from build123d import *

# Parameters (mm, degrees)
BOSS_EXTRUDE1_DEPTH = 6


with BuildPart() as part:
    # Sketch1 → Boss-Extrude1 (new body)
    with BuildSketch(Plane.XY):
        with BuildLine():
            Line((0, 0), (0, 100))
            Line((0, 100), (0, 116.099356626))
            ThreePointArc((0, 116.099356626), (5.566363801, 126.764301673), (17.498623517, 128.296175326))
            Line((17.498623517, 128.296175326), (69.668134054, 109.054191593))
            ThreePointArc((69.668134054, 109.054191593), (74.638707981, 99.521504918), (65.633362838, 93.649326508))
            Line((65.633362838, 93.649326508), (38.741282829, 97.960661065))
            ThreePointArc((38.741282829, 97.960661065), (29.863968579, 95.470560576), (25.999999999, 87.099356626))
            Line((25.999999999, 87.099356626), (25.999999999, -325.14105767))
            ThreePointArc((25.999999999, -325.14105767), (26.999999698, -326.141057369), (27.999999397, -325.14105767))
            Line((27.999999397, -325.14105767), (27.999999397, -295.628663382))
            Line((27.999999397, -295.628663382), (29.999999399, -295.628663382))
            Line((29.999999399, -295.628663382), (29.999999399, -325.14105767))
            ThreePointArc((29.999999399, -325.14105767), (26.999999699, -328.14105737), (23.999999999, -325.14105767))
            Line((23.999999999, -325.14105767), (23.999999999, 87.099356626))
            ThreePointArc((23.999999999, 87.099356626), (28.56650832, 96.992597657), (39.057879707, 99.93544369))
            Line((39.057879707, 99.93544369), (65.949959716, 95.624109133))
            ThreePointArc((65.949959716, 95.624109133), (72.703968573, 100.02824294), (68.976038128, 107.177757947))
            Line((68.976038128, 107.177757947), (16.806527591, 126.41974168))
            ThreePointArc((16.806527591, 126.41974168), (6.710000139, 125.123540896), (2, 116.099356626))
            Line((2, 116.099356626), (2, 100))
            Line((2, 100), (2, 0))
            Line((2, 0), (2, -733.96669053))
            ThreePointArc((2, -733.96669053), (13, -744.96669053), (24, -733.96669053))
            Line((24, -733.96669053), (24, -340.488878189))
            ThreePointArc((24, -340.488878189), (26.9999997, -337.488878489), (29.9999994, -340.488878189))
            Line((29.9999994, -340.488878189), (29.9999994, -370.001272476))
            Line((29.9999994, -370.001272476), (27.999999398, -370.001272476))
            Line((27.999999398, -370.001272476), (27.999999398, -340.488878189))
            ThreePointArc((27.999999398, -340.488878189), (26.999999699, -339.48887849), (26, -340.488878189))
            Line((26, -340.488878189), (26, -733.96669053))
            ThreePointArc((26, -733.96669053), (13, -746.96669053), (0, -733.96669053))
            Line((0, -733.96669053), (0, 0))
        make_face()
    extrude(amount=BOSS_EXTRUDE1_DEPTH)


solid = part.part
The listing builds one solid part. Answer for the finished solid, in the listing's coordinates (mm). Give positions to 0.01 mm unless a question says otherwise; leave off trailing zeros. Write each loop counter-clockwise with the first axis right and the second up, starting at its lowest first coordinate (ties: lowest second). Pieces come first, ordered by that corner, then holes. Notation, with made-up numbers: (20, 4) - (63, 4) arc R14 cw to (63, 13) - close; hole circle Ø5 at (-12.75, 15). An arc over 180 degrees is marked (long way). One line per question, with ' | ' between items. Start each with the question number.
1. Section C-C, the plane z = 3.95 is taken. Determine the outline of the cut face in (x, y), then the cut area to 3 significant figures.
2. Section A-A, the plane y = -629.5 is taken. Determine the outline of the cut face in (x, z).
3. Given P1, Ø3, axis at y = -354.5, z = 3, coming from the +X side; P2, Ø1.8, axis at y = -96, z = 4, coming from the +X side; P3, Ø2, axis at x = 29, z = 1.5, coming from the -Y side; P4, Ø12, axis at x = 16, y = -447, coming from the -Z side, each flat-ended and moving along its own axis, determine where each tip first touches the part or whether it passes through.
4. Determine the mould class of faces 1 (the face through (1.6, -274.4, 0)), 2 (the face through (43.256, 116.664, 2.958)), 3 (the face through (43.22, 118.81, 2.96)) for opening direction Y: +Y half, -Y half, draft (parallel to the pull), parting line (faces both ways), or undercut.
5. Section B-B, the plane x = 56 is taken. Determine the outline of the cut face in (y, z).
6. Straight lines are drawn through the part: line 1 (X direction, y = -309, z = 3.5); line 2 (X direction, y = -561.5, z = 3.3); line 3 (Y direction, x = 28.5, z = 1.5). For each, find the intervals that lie inside material, in ascending order.
Result:
1) outline: (0, -733.97) arc R13 ccw to (26, -733.97) - (26, -340.49) arc R1 cw to (28, -340.49) - (28, -370) - (30, -370) - (30, -340.49) arc R3 ccw to (24, -340.49) - (24, -733.97) arc R11 cw to (2, -733.97) - (2, 116.1) arc R11 cw to (16.81, 126.42) - (68.98, 107.18) arc R6 cw to (65.95, 95.62) - (39.06, 99.94) arc R13 ccw to (24, 87.1) - (24, -325.14) arc R3 ccw to (30, -325.14) - (30, -295.63) - (28, -295.63) - (28, -325.14) arc R1 cw to (26, -325.14) - (26, 87.1) arc R11 cw to (38.74, 97.96) - (65.63, 93.65) arc R8 ccw to (69.67, 109.05) - (17.5, 128.3) arc R13 ccw to (0, 116.1) - close | area: 3,820 mm2
2) outline: (0, 0) - (2, 0) - (2, 6) - (0, 6) - close; (24, 0) - (26, 0) - (26, 6) - (24, 6) - close
3) P1: stops at x = 30 | P2: stops at x = 26 | P3: stops at y = -370 | P4: passes through
4) face 1: draft | face 2: undercut | face 3: +Y half
5) outline: (95.19, 0) - (97.22, 0) - (97.22, 6) - (95.19, 6) - close; (111.96, 0) - (114.1, 0) - (114.1, 6) - (111.96, 6) - close
6) line 1: x = 0 to 2, 24 to 26, 28 to 30 | line 2: x = 0 to 2, 24 to 26 | line 3: y = -370 to -337.89, -327.74 to -295.63, 94.08 to 96.94, 122.11 to 124.24
